Design review of the part shown in the three views and the two pictorial views. Dimensions are in mm from the part's minimum x, y and z. Give positions to 0.01 mm unless a question says otherwise; leave off trailing zeros. Loops run counter-clockwise (first coordinate to the right, second up) from the corner with the lowest first, then second, coordinate; pieces in that order, holes last. Notation, with made-up numbers: (71, -36.75) -> (90, -36.75) arc R19 cw to (90, -16.75) -> close; hole circle Ø9 at (39.5, 89). An arc over 180 degrees is marked (long way). Answer as CSV lines item,"result".
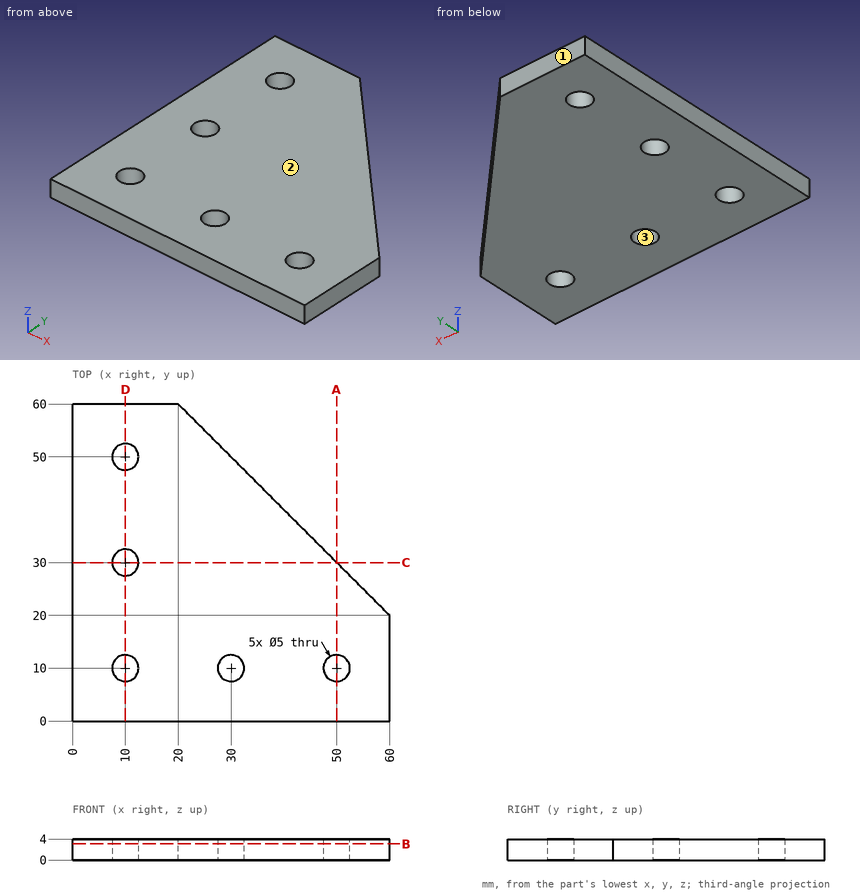
Q1. The part is to be moulded in two halves that separate along Y. For the marked faces 1, 2 and 3, say which applies: pulls with the +Y half, pulls with the -Y half, needs draft (parallel to the pull), parting line crosses it, or undercut.
Filled sheet:
face 1,"pulls with the +Y half"
face 2,"needs draft"
face 3,"undercut"
Q2. To check wall thickness, follow probe 1 along Y at (x, z) = (10, 1.95); probe 2 along X at (y, z) = (11.5, 1.15); probe 3 along Y at (x, z) = (30, 1.8). State the ranges of each line that lie inside material, in increasing order. Write a range as from..to.
Filled sheet:
probe 1,"y = 0..7.5, 12.5..27.5, 32.5..47.5, 52.5..60"
probe 2,"x = 0..8, 12..28, 32..48, 52..60"
probe 3,"y = 0..7.5, 12.5..50"
Q3. We need section B-B, the plane z = 3.1. State the section outline as (x, y) points.
Filled sheet:
outline,"(0, 0) -> (60, 0) -> (60, 20) -> (20, 60) -> (0, 60) -> close; hole circle Ø5 at (10, 10); hole circle Ø5 at (10, 30); hole circle Ø5 at (10, 50); hole circle Ø5 at (30, 10); hole circle Ø5 at (50, 10)"
Q4. We need section C-C, the plane y = 30. State the section outline as (x, z) points, and give its area (3 significant figures).
Filled sheet:
outline,"(0, 0) -> (7.5, 0) -> (7.5, 4) -> (0, 4) -> close; (12.5, 0) -> (50, 0) -> (50, 4) -> (12.5, 4) -> close"
area,"180 mm^2"
Q5. We need section D-D, the plane x = 10. State the section outline as (y, z) points, and give its area (3 significant figures).
Filled sheet:
outline,"(0, 0) -> (7.5, 0) -> (7.5, 4) -> (0, 4) -> close; (12.5, 0) -> (27.5, 0) -> (27.5, 4) -> (12.5, 4) -> close; (32.5, 0) -> (47.5, 0) -> (47.5, 4) -> (32.5, 4) -> close; (52.5, 0) -> (60, 0) -> (60, 4) -> (52.5, 4) -> close"
area,"180 mm^2"
Q6. We need section A-A, the plane x = 50. State the section outline as (y, z) points.
Filled sheet:
outline,"(0, 0) -> (7.5, 0) -> (7.5, 4) -> (0, 4) -> close; (12.5, 0) -> (30, 0) -> (30, 4) -> (12.5, 4) -> close"
